from build123d import *

# Parameters (mm, degrees)
SKETCH1_R            = 12.1
BOSS_EXTRUDE1_DEPTH  = 3
BOSS_EXTRUDE2_DEPTH  = 3
BOSS_EXTRUDE3_DEPTH  = 3
BOSS_EXTRUDE4_DEPTH  = 3
BOSS_EXTRUDE5_DEPTH  = 3
BOSS_EXTRUDE6_DEPTH  = 3
BOSS_EXTRUDE7_DEPTH  = 3
BOSS_EXTRUDE8_DEPTH  = 3
BOSS_EXTRUDE9_DEPTH  = 3
BOSS_EXTRUDE10_DEPTH = 3
BOSS_EXTRUDE11_DEPTH = 3
BOSS_EXTRUDE12_DEPTH = 3
BOSS_EXTRUDE13_DEPTH = 3
BOSS_EXTRUDE14_DEPTH = 3
BOSS_EXTRUDE15_DEPTH = 3
BOSS_EXTRUDE16_DEPTH = 3
BOSS_EXTRUDE17_DEPTH = 3
BOSS_EXTRUDE18_DEPTH = 3
BOSS_EXTRUDE19_DEPTH = 3
BOSS_EXTRUDE20_DEPTH = 3
BOSS_EXTRUDE21_DEPTH = 3
BOSS_EXTRUDE22_DEPTH = 3
BOSS_EXTRUDE23_DEPTH = 3
BOSS_EXTRUDE24_DEPTH = 3
BOSS_EXTRUDE25_DEPTH = 3
SKETCH26_W           = 31
SKETCH26_H           = 6
BOSS_EXTRUDE26_DEPTH = 3
SKETCH27_R           = 4
BOSS_EXTRUDE27_DEPTH = 3


with BuildPart() as part:
    # Sketch1 → Boss-Extrude1 (new body)
    with BuildSketch(Plane.XY):
        Circle(SKETCH1_R)
    extrude(amount=BOSS_EXTRUDE1_DEPTH)

    # Sketch2 → Boss-Extrude2 (add)
    with BuildSketch(Plane.XY):
        Polygon((12.079935981, -0.696524726), (14.645079707, -0.379658233), (14.645079707, 0.379658233), (12.079935981, 0.696524726), align=None)
    extrude(amount=BOSS_EXTRUDE2_DEPTH)

    # Sketch3 → Boss-Extrude3 (add)
    with BuildSketch(Plane.XY):
        Polygon((11.848596009, 2.453726274), (14.244323498, 3.423703853), (14.244323498, 4.157147238), (11.490982299, 3.790425545), align=None)
    extrude(amount=BOSS_EXTRUDE3_DEPTH)

    # Sketch4 → Boss-Extrude4 (add)
    with BuildSketch(Plane.XY):
        Polygon((10.809793799, 5.436759883), (12.872840183, 6.993746179), (12.418878698, 7.595256676), (10.113269073, 6.643176098), align=None)
    extrude(amount=BOSS_EXTRUDE4_DEPTH)

    # Sketch5 → Boss-Extrude5 (add)
    with BuildSketch(Plane.XY):
        Polygon((9.034322006, 8.049287291), (10.624094083, 10.087176261), (9.829208044, 10.707272668), (8.182693208, 8.913671065), align=None)
    extrude(amount=BOSS_EXTRUDE5_DEPTH)

    # Sketch6 → Boss-Extrude6 (add)
    with BuildSketch(Plane.XY):
        Polygon((6.643176098, 10.113269073), (7.651333528, 12.49318195), (7.147254813, 12.706715272), (5.436759883, 10.809793799), align=None)
    extrude(amount=BOSS_EXTRUDE6_DEPTH)

    # Sketch7 → Boss-Extrude7 (add)
    with BuildSketch(Plane.XY):
        Polygon((3.799308717, 11.488048279), (4.157147238, 14.047797936), (3.423703853, 14.047797936), (2.453726274, 11.848596009), align=None)
    extrude(amount=BOSS_EXTRUDE7_DEPTH)

    # Sketch8 → Boss-Extrude8 (add)
    with BuildSketch(Plane.XY):
        Polygon((0.696524726, 12.079935981), (0.379658233, 14.645079707), (-0.379658233, 14.645079707), (-0.696524726, 12.079935981), align=None)
    extrude(amount=BOSS_EXTRUDE8_DEPTH)

    # Sketch9 → Boss-Extrude9 (add)
    with BuildSketch(Plane.XY):
        Polygon((-2.453726274, 11.848596009), (-3.423703853, 14.244323498), (-4.157147238, 14.244323498), (-3.790425545, 11.490982299), align=None)
    extrude(amount=BOSS_EXTRUDE9_DEPTH)

    # Sketch10 → Boss-Extrude10 (add)
    with BuildSketch(Plane.XY):
        Polygon((-5.436759883, 10.809793799), (-6.993746179, 12.872840183), (-7.595256676, 12.418878698), (-6.643176098, 10.113269073), align=None)
    extrude(amount=BOSS_EXTRUDE10_DEPTH)

    # Sketch11 → Boss-Extrude11 (add)
    with BuildSketch(Plane.XY):
        Polygon((-8.049287291, 9.034322006), (-10.087176261, 10.624094083), (-10.707272668, 9.829208044), (-8.913671065, 8.182693208), align=None)
    extrude(amount=BOSS_EXTRUDE11_DEPTH)

    # Sketch12 → Boss-Extrude12 (add)
    with BuildSketch(Plane.XY):
        Polygon((-10.113269073, 6.643176098), (-12.49318195, 7.651333528), (-12.706715272, 7.147254813), (-10.809793799, 5.436759883), align=None)
    extrude(amount=BOSS_EXTRUDE12_DEPTH)

    # Sketch13 → Boss-Extrude13 (add)
    with BuildSketch(Plane.XY):
        Polygon((-11.488048279, 3.799308717), (-14.047797936, 4.157147238), (-14.047797936, 3.423703853), (-11.848596009, 2.453726274), align=None)
    extrude(amount=BOSS_EXTRUDE13_DEPTH)

    # Sketch14 → Boss-Extrude14 (add)
    with BuildSketch(Plane.XY):
        Polygon((-12.079935981, 0.696524726), (-14.645079707, 0.379658233), (-14.645079707, -0.379658233), (-12.079935981, -0.696524726), align=None)
    extrude(amount=BOSS_EXTRUDE14_DEPTH)

    # Sketch15 → Boss-Extrude15 (add)
    with BuildSketch(Plane.XY):
        Polygon((-11.848596009, -2.453726274), (-14.244323498, -3.423703853), (-14.244323498, -4.157147238), (-11.490982299, -3.790425545), align=None)
    extrude(amount=BOSS_EXTRUDE15_DEPTH)

    # Sketch16 → Boss-Extrude16 (add)
    with BuildSketch(Plane.XY):
        Polygon((-10.809793799, -5.436759883), (-12.872840183, -6.993746179), (-12.418878698, -7.595256676), (-10.113269073, -6.643176098), align=None)
    extrude(amount=BOSS_EXTRUDE16_DEPTH)

    # Sketch17 → Boss-Extrude17 (add)
    with BuildSketch(Plane.XY):
        Polygon((-9.034322006, -8.049287291), (-10.624094083, -10.087176261), (-9.829208044, -10.707272668), (-8.182693208, -8.913671065), align=None)
    extrude(amount=BOSS_EXTRUDE17_DEPTH)

    # Sketch18 → Boss-Extrude18 (add)
    with BuildSketch(Plane.XY):
        Polygon((-6.643176098, -10.113269073), (-7.651333528, -12.49318195), (-7.147254813, -12.706715272), (-5.436759883, -10.809793799), align=None)
    extrude(amount=BOSS_EXTRUDE18_DEPTH)

    # Sketch19 → Boss-Extrude19 (add)
    with BuildSketch(Plane.XY):
        Polygon((-3.799308717, -11.488048279), (-4.157147238, -14.047797936), (-3.423703853, -14.047797936), (-2.453726274, -11.848596009), align=None)
    extrude(amount=BOSS_EXTRUDE19_DEPTH)

    # Sketch20 → Boss-Extrude20 (add)
    with BuildSketch(Plane.XY):
        Polygon((-0.696524726, -12.079935981), (-0.696524726, -14.645079707), (0.379658233, -14.645079707), (0.379658233, -12.09404232), align=None)
    extrude(amount=BOSS_EXTRUDE20_DEPTH)

    # Sketch21 → Boss-Extrude21 (add)
    with BuildSketch(Plane.XY):
        Polygon((2.453726274, -11.848596009), (3.423703853, -14.244323498), (4.157147238, -14.244323498), (3.790425545, -11.490982299), align=None)
    extrude(amount=BOSS_EXTRUDE21_DEPTH)

    # Sketch22 → Boss-Extrude22 (add)
    with BuildSketch(Plane.XY):
        Polygon((5.436759883, -10.809793799), (6.993746179, -12.872840183), (7.595256676, -12.418878698), (6.643176098, -10.113269073), align=None)
    extrude(amount=BOSS_EXTRUDE22_DEPTH)

    # Sketch23 → Boss-Extrude23 (add)
    with BuildSketch(Plane.XY):
        Polygon((8.049287291, -9.034322006), (9.863117815, -10.848152529), (10.770033076, -9.941237267), (8.89125817, -8.207041376), align=None)
    extrude(amount=BOSS_EXTRUDE23_DEPTH)

    # Sketch24 → Boss-Extrude24 (add)
    with BuildSketch(Plane.XY):
        Polygon((10.113269073, -6.643176098), (12.49318195, -7.651333528), (12.706715272, -7.147254813), (10.809793799, -5.436759883), align=None)
    extrude(amount=BOSS_EXTRUDE24_DEPTH)

    # Sketch25 → Boss-Extrude25 (add)
    with BuildSketch(Plane.XY):
        Polygon((11.488048279, -3.799308717), (14.047797936, -4.157147238), (14.047797936, -3.423703853), (11.848596009, -2.453726274), align=None)
    extrude(amount=BOSS_EXTRUDE25_DEPTH)

    # Sketch26 → Boss-Extrude26 (add)
    with BuildSketch(Plane.XY):
        with Locations((-15.5, 0)):
            Rectangle(SKETCH26_W, SKETCH26_H)
    extrude(amount=BOSS_EXTRUDE26_DEPTH)

    # Sketch27 → Boss-Extrude27 (add)
    with BuildSketch(Plane.XY):
        with Locations((-31, 0)):
            Circle(SKETCH27_R)
    extrude(amount=BOSS_EXTRUDE27_DEPTH)


solid = part.part
Here's how the part is built. I have some questions about the finished solid (model axes, mm). A direction names the side the tool comes from. Coordinates: 2 decimals unless noted, no trailing zeros. Order: outer loops, then holes, each group sorted by start corner. A loop starts at its lowest first (then second) coordinate and runs counter-clockwise, first axis right, second up. Notation, with made-up numbers: (36.5, 11) -> (90.5, 11) arc R22 cw to (90.5, 33) -> close; hole circle Ø11 at (87, 34.5). An arc over 180 degrees is marked (long way). Answer in a Markdown table with one row per item.
(1) Thinking about a two-plate mould opening in Y: for faces 1 (the face through (13.38, 0.536, 1.479)), 2 (the face through (1.407, -12.018, 1.479)), 3 (the face through (1.592, 11.995, 1.479)), which applies, +Y half, -Y half, draft (parallel to the pull), parting line (faces both ways), or undercut?
Answer key:
| item | result |
|---|---|
| face 1 | undercut |
| face 2 | -Y half |
| face 3 | +Y half |
(2) I want a section at A-A on x = -31. List the corners of the cut face in (y, z) for me.
Answer key:
| item | result |
|---|---|
| outline | (-4, 0) -> (4, 0) -> (4, 3) -> (-4, 3) -> close |
(3) On a 3-axis mill with a long thin cutter (end or side, diameter ignored), from which of +Z, -Z, +X, -X, +Y, -Y can I reach the whole of each face in a straight line? I mean faces 4 (the face through (-6.3, -11.77, 1.48)), 5 (the face through (12.887, 3.976, 1.479)), 6 (the face through (13.03, 2.93, 1.48)), 7 (the face through (-5, 0, 3)), 8 (the face through (-6.204, 11.827, 1.479)). Say none if no direction works.
Answer key:
| item | result |
|---|---|
| face 4 | +Z, -Z, -Y |
| face 5 | +Z, -Z |
| face 6 | +Z, -Z, +X |
| face 7 | +Z, +X, -X, +Y, -Y |
| face 8 | +Z, -Z, +Y |
(4) Please list where these lines run through material, in increasing order: probe 1 along X at (y, z) = (12.75, 1.75); probe 2 along X at (y, z) = (-12.25, 0.65); probe 3 along X at (y, z) = (10, 2.2).
Answer key:
| item | result |
|---|---|
| probe 1 | -7.16 to -6.9, -3.96 to -2.82, -0.61 to 0.61, 2.85 to 3.98 |
| probe 2 | -7.55 to -6.74, -3.91 to -2.63, -0.7 to 0.38, 2.62 to 3.89, 6.52 to 7.53 |
| probe 3 | -10.57 to -9.29, -6.81 to 6.81, 9.18 to 10.56 |
(5) I want a section at B-B on x = -26. List the corners of the cut face in (y, z) for me.
Answer key:
| item | result |
|---|---|
| outline | (-3, 0) -> (3, 0) -> (3, 3) -> (-3, 3) -> close |
(6) Will these pins go through, and if not, where does the flat tip stop? pin 1 Ø1.5 at (x, z) = (-5, 1.5) entering from -Y; pin 2 Ø1 at (y, z) = (-6, 1) entering from +X; pin 3 Ø0.8 at (x, z) = (3.5, 1.5) entering from +Y; pin 4 Ø10 at (x, y) = (9, -11.5) entering from -Z.
Answer key:
| item | result |
|---|---|
| pin 1 | y = -11.33 |
| pin 2 | x = 11.99 |
| pin 3 | y = 14.05 |
| pin 4 | z = 0 |
